Input: part model. Units: mm. Frame: model coordinates. Round coordinates to 2 decimals unless told otherwise and drop trailing zeros. Loops run counter-clockwise (first coordinate to the right, second up) from the corner with the lowest first, then second, coordinate; pieces in that order, holes last. Notation, with made-up numbers: (-17.75, 25) - (6.25, 25) arc R20 cw to (6.25, 58) - close; hole circle Ø5 at (42, 11.25). An arc over 180 degrees is marked (long way). One line per question, with ' | ' between items. Start each with the question number.
Item 1: Section B-B, the plane y = -56.5. Return loops of the section in (x, z), plus the area to 3 significant figures.
Item 2: Section C-C, the plane z = 0.75. Give the number of separate pieces and of enclosed holes in the cut face, plus the area to 3 significant figures.
Item 3: Section A-A, the plane x = 16.5. Return loops of the section in (y, z).
Item 4: First-contact query: pin 1 (2 mm diameter, centred on x = -7.94, y = -72.59, fed in from +Z); pin 2 (0.6 mm diameter, centred on x = 31, z = 1, fed in from -Y); pin 3 (1 mm diameter, centred on x = 19.5, z = 0.5, fed in from +Y). Flat tips, straight axial feed; report the tip coordinate or a pass-through.
Item 5: Material intervals for line 1 along Y through (x, z) = (-7.5, 0.65); line 2 along X through (y, z) = (-45.5, 1.2); line 3 along X through (y, z) = (-73, 1.55), sorted ascending.
```python
from build123d import *

# Parameters (mm, degrees)
SKETCH_1_R          = 2.1
EXTRUDE_1_DEPTH     = 2
SKETCH_2_W          = 35
SKETCH_2_H          = 2
EXTRUDE_2_DEPTH     = 30
SKETCH_4_W          = 35
SKETCH_4_H          = 3
CUT_EXTRUDE_2_DEPTH = 10
SKETCH_5_R          = 1.25
CUT_EXTRUDE_3_DEPTH = 10


with BuildPart() as part:
    # 草图1 → 凸台-拉伸1 (new body)
    with BuildSketch(Plane.XY):
        with BuildLine():
            Line((-33.941138155, 25.010321846), (-33.941138155, 3.010321846))
            ThreePointArc((-33.941138155, 3.010321846), (-33.062458498, 0.889001502), (-30.941138155, 0.010321846))
            Line((-30.941138155, 0.010321846), (-27.683778842, 0.010321846))
            ThreePointArc((-27.683778842, 0.010321846), (-26.535728545, -0.218039556), (-25.562458498, -0.86835781))
            Line((-25.562458498, -0.86835781), (-17.319817811, -9.110998498))
            ThreePointArc((-17.319817811, -9.110998498), (-16.669499557, -10.084268544), (-16.441138155, -11.232318841))
            Line((-16.441138155, -11.232318841), (-16.441138155, -59.216175462))
            Line((-16.441138155, -59.216175462), (18.558861845, -59.216175462))
            Line((18.558861845, -59.216175462), (18.558861845, -11.232318841))
            ThreePointArc((18.558861845, -11.232318841), (18.787223248, -10.084268544), (19.437541502, -9.110998498))
            Line((19.437541502, -9.110998498), (27.680182189, -0.86835781))
            ThreePointArc((27.680182189, -0.86835781), (28.653452235, -0.218039556), (29.801502532, 0.010321846))
            Line((29.801502532, 0.010321846), (33.058861845, 0.010321846))
            ThreePointArc((33.058861845, 0.010321846), (35.180182189, 0.889001502), (36.058861845, 3.010321846))
            Line((36.058861845, 3.010321846), (36.058861845, 25.010321846))
            ThreePointArc((36.058861845, 25.010321846), (1.058861845, 60.010321846), (-33.941138155, 25.010321846))
        make_face()
        with Locations((26.173598555, 10.510321846)):
            Circle(SKETCH_1_R, mode=Mode.SUBTRACT)
        with Locations((-24.055874865, 10.510321846)):
            Circle(SKETCH_1_R, mode=Mode.SUBTRACT)
        with Locations((1.058861845, 54.010321846)):
            Circle(SKETCH_1_R, mode=Mode.SUBTRACT)
        with BuildLine():
            Line((13.630967923, 33.192140028), (4.830493669, 46.714867301))
            ThreePointArc((4.830493669, 46.714867301), (1.058861845, 48.760321846), (-2.712769978, 46.714867301))
            Line((-2.712769978, 46.714867301), (-11.513244233, 33.192140028))
            ThreePointArc((-11.513244233, 33.192140028), (-11.931519212, 32.510321846), (-12.312853589, 31.807175998))
            Line((-12.312853589, 31.807175998), (-19.623641808, 17.424378092))
            ThreePointArc((-19.623641808, 17.424378092), (-19.509241495, 13.135321846), (-15.852009984, 10.891720146))
            Line((-15.852009984, 10.891720146), (0.25925249, 10.031649512))
            ThreePointArc((0.25925249, 10.031649512), (1.058861845, 10.010321846), (1.858471201, 10.031649512))
            Line((1.858471201, 10.031649512), (17.969733675, 10.891720146))
            ThreePointArc((17.969733675, 10.891720146), (21.626965185, 13.135321846), (21.741365498, 17.424378092))
            Line((21.741365498, 17.424378092), (14.430577279, 31.807175998))
            ThreePointArc((14.430577279, 31.807175998), (14.049242902, 32.510321846), (13.630967923, 33.192140028))
        make_face(mode=Mode.SUBTRACT)
    extrude(amount=EXTRUDE_1_DEPTH)

    # 草图2 → 凸台-拉伸2 (add)
    with BuildSketch(Plane.XZ.offset(59.216175462)):
        with Locations((1.058861845, 1)):
            Rectangle(SKETCH_2_W, SKETCH_2_H)
    extrude(amount=EXTRUDE_2_DEPTH)

    # 草图4 → 切除-拉伸2 (cut)
    with BuildSketch(Plane.XY.offset(2)):
        with Locations((1.058861845, -87.716175462)):
            Rectangle(SKETCH_4_W, SKETCH_4_H)
    extrude(amount=-CUT_EXTRUDE_2_DEPTH, mode=Mode.SUBTRACT)

    # 草图5 → 切除-拉伸3 (cut)
    with BuildSketch(Plane.XY.offset(2)):
        with Locations((10.058861845, -27.388786859)):
            Circle(SKETCH_5_R)
        with Locations((-7.941138155, -27.388786859)):
            Circle(SKETCH_5_R)
        with Locations((-7.941138155, -72.588786859)):
            Circle(SKETCH_5_R)
        with Locations((10.058861845, -72.588786859)):
            Circle(SKETCH_5_R)
    extrude(amount=-CUT_EXTRUDE_3_DEPTH, mode=Mode.SUBTRACT)


solid = part.part
```
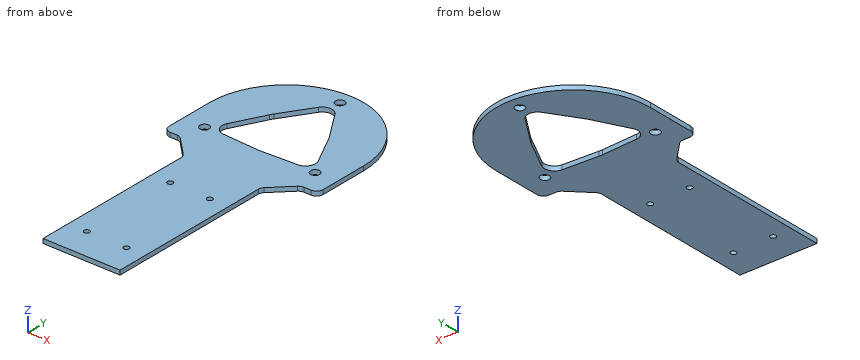
Return value:
1) outline: (-16.44, 0) - (18.56, 0) - (18.56, 2) - (-16.44, 2) - close | area: 70.0 mm2
2) separate pieces: 1 | enclosed holes: 8 | area: 5,690 mm2
3) outline: (-86.22, 0) - (10.81, 0) - (10.81, 2) - (-86.22, 2) - close; (27.74, 0) - (56.42, 0) - (56.42, 2) - (27.74, 2) - close
4) pin 1: through | pin 2: y = 0.01 | pin 3: y = 55.06
5) line 1: -86.22 to -73.76, -71.42 to -28.56, -26.22 to 10.45, 39.36 to 58.95 | line 2: -16.44 to 18.56 | line 3: -16.44 to -9.12, -6.76 to 8.88, 11.24 to 18.56
